Source: CAD feature listing. Evaluate the final solid. Frame: model axes, mm. A direction names the side the tool comes from. Coordinates: 2 decimals unless noted, no trailing zeros. Order: outer loops, then holes, each group sorted by start corner. A loop starts at its lowest first (then second) coordinate and runs counter-clockwise, first axis right, second up.
```python
from build123d import *

# Parameters (mm, degrees)
SKETCH1_R           = 10
SKETCH1_R_2         = 1.25
BOSS_EXTRUDE1_DEPTH = 5
BOSS_EXTRUDE2_DEPTH = 5
SKETCH3_W           = 10
SKETCH3_H           = 10
BOSS_EXTRUDE3_DEPTH = 20
SKETCH4_R           = 3
CUT_EXTRUDE1_DEPTH  = 6
CHAMFER1_SIZE       = 3
SKETCH5_W           = 6
SKETCH5_H           = 5
CUT_EXTRUDE2_DEPTH  = 3


with BuildPart() as part:
    # Sketch1 → Boss-Extrude1 (new body)
    with BuildSketch(Plane(origin=(0, 0, 0), x_dir=(1, 0, 0), z_dir=(0, 1, 0))):
        with Locations(Location((0, 0, 0), (0, 0, 270))):
            Circle(SKETCH1_R)
        with Locations(Location((0, 7, 0), (0, 0, 270))):
            Circle(SKETCH1_R_2, mode=Mode.SUBTRACT)
        with Locations(Location((7, 0, 0), (0, 0, 270))):
            Circle(SKETCH1_R_2, mode=Mode.SUBTRACT)
        with Locations(Location((0, -7, 0), (0, 0, 270))):
            Circle(SKETCH1_R_2, mode=Mode.SUBTRACT)
        with Locations(Location((-7, 0, 0), (0, 0, 270))):
            Circle(SKETCH1_R_2, mode=Mode.SUBTRACT)
    extrude(amount=BOSS_EXTRUDE1_DEPTH)

    # Sketch2 → Boss-Extrude2 (add)
    with BuildSketch(Plane(origin=(0, 0, 0), x_dir=(1, 0, 0), z_dir=(0, 1, 0))):
        with BuildLine():
            Line((0, 10), (105, 10))
            Line((105, 10), (105, -10))
            Line((105, -10), (0, -10))
            ThreePointArc((0, -10), (10, 0), (0, 10))
        make_face()
    extrude(amount=BOSS_EXTRUDE2_DEPTH)

    # Sketch3 → Boss-Extrude3 (add)
    with BuildSketch(Plane(origin=(0, 0, -10), x_dir=(-1, 0, 0), z_dir=(0, 0, -1))):
        with Locations((-100, 5)):
            Rectangle(SKETCH3_W, SKETCH3_H)
    extrude(amount=-BOSS_EXTRUDE3_DEPTH)

    # Sketch4 → Cut-Extrude1 (cut)
    with BuildSketch(Plane(origin=(0, 0, -10), x_dir=(-1, 0, 0), z_dir=(0, 0, -1))):
        with Locations((-100, 5)):
            Circle(SKETCH4_R)
    extrude(amount=-CUT_EXTRUDE1_DEPTH, mode=Mode.SUBTRACT)

    # Chamfer1
    chamfer1_edges = [part.edges().sort_by_distance(p)[0] for p in [
        (103, 5, -4),
    ]]
    chamfer(chamfer1_edges, length=CHAMFER1_SIZE)

    # Sketch5 → Cut-Extrude2 (cut)
    with BuildSketch(Plane(origin=(0, 0, -10), x_dir=(-1, 0, 0), z_dir=(0, 0, -1))):
        with Locations((-100, 2.5)):
            Rectangle(SKETCH5_W, SKETCH5_H)
    extrude(amount=-CUT_EXTRUDE2_DEPTH, mode=Mode.SUBTRACT)


solid = part.part
```
Q1. Section query B-B on z = 7. Output: boundary loops of the cut face in (x, y), plus the area to 3 significant figures.
Solutions:
outline: (-7.14, 0) - (-1.25, 0) - (-1.25, 5) - (-7.14, 5) - close; (1.25, 0) - (105, 0) - (105, 10) - (95, 10) - (95, 5) - (1.25, 5) - close
area: 598 mm2
Q2. Material intervals for line 1 along X through (y, z) = (3.25, 0); line 2 along X through (y, z) = (3.5, -1); line 3 along Y through (x, z) = (72, -1.75), sorted ascending.
Solutions:
line 1: x = -10 to -8.25, -5.75 to 5.75, 8.25 to 105
line 2: x = -9.95 to -7.75, -6.25 to 6.25, 7.75 to 105
line 3: y = 0 to 5
Q3. Pull-direction query (Z, two-part tool) for faces 4 (the cylindrical face through (0.05, 2.46, 5.75)), 5 (the flat face through (100, 10, 0)), 6 (the conical face through (99, 5, -5)); classes: pulls with the +Z half, pulls with the -Z half, needs draft (parallel to the pull), parting line crosses it, or undercut.
Solutions:
face 4: undercut
face 5: needs draft
face 6: pulls with the -Z half
Q4. Section query A-A on x = 7. Output: boundary loops of the cut face in (y, z), plus the area to 3 significant figures.
Solutions:
outline: (0, -10) - (5, -10) - (5, -1.25) - (0, -1.25) - close; (0, 1.25) - (5, 1.25) - (5, 10) - (0, 10) - close
area: 87.5 mm2
Q5. Pin query (flat end, axial travel): P1, Ø1.5, axis at y = 8, z = -1.5, coming from the -X side; P2, Ø3, axis at x = 66, z = 7, coming from the +Y side; P3, Ø3.5, axis at y = 3.5, z = -9, coming from the -X side. Return the tip coordinate at first contact, or that it passes through.
Solutions:
P1: stops at x = 95
P2: stops at y = 5
P3: stops at x = -6.89
Q6. Section query D-D on z = -2.5. Output: boundary loops of the cut face in (x, y).
Solutions:
outline: (-9.68, 0) - (105, 0) - (105, 10) - (95, 10) - (95, 5) - (-9.68, 5) - close
Q7. Set-up query: faces 1 (the flat face through (95, 7, 0)), 2 (the flat face through (97, 2, -9)), 3 (the cylindrical face through (0.05, 2.46, -8.25)). Return all of +Z, -Z, +X, -X, +Y, -Y with unobstructed straight access to the full face (end or side cutting, diameter ignored); none if empty.
Solutions:
face 1: +Z, -Z, -X, +Y
face 2: -Z, -Y
face 3: +Y, -Y
Q8. Section query C-C on x = -7. Output: boundary loops of the cut face in (y, z).
Solutions:
outline: (0, -7.14) - (5, -7.14) - (5, -1.25) - (0, -1.25) - close; (0, 1.25) - (5, 1.25) - (5, 7.14) - (0, 7.14) - close
